Check sheet for the modelled part. Datum: model origin and axes. Units: mm. A direction names the side the tool comes from. Round coordinates to 2 decimals unless told otherwise and drop trailing zeros. Order: outer loops, then holes, each group sorted by start corner. A loop starts at its lowest first (then second) coordinate and runs counter-clockwise, first axis right, second up.
```python
from build123d import *

# Parameters (mm, degrees)
SKETCH1_W           = 26
SKETCH1_H           = 42
BOSS_EXTRUDE1_DEPTH = 16
SHELL1_T            = -2
SKETCH2_R           = 3.8
SKETCH2_R_2         = 1.8
BOSS_EXTRUDE2_DEPTH = 3
CUT_EXTRUDE2_START  = -2
SKETCH2_2_R         = 1.8
CUT_EXTRUDE2_DEPTH  = 2
SKETCH4_W           = 8
SKETCH4_H           = 10.725495138
CUT_EXTRUDE3_DEPTH  = 2
SKETCH5_W           = 6
SKETCH5_H           = 8.708980209
CUT_EXTRUDE4_DEPTH  = 2


with BuildPart() as part:
    # Sketch1 → Boss-Extrude1 (new body)
    with BuildSketch(Plane.XY):
        Rectangle(SKETCH1_W, SKETCH1_H)
    extrude(amount=BOSS_EXTRUDE1_DEPTH)

    # Shell1
    shell1_openings = [part.faces().sort_by_distance(p)[0] for p in [
        (0, 0, 16),
    ]]
    offset(amount=SHELL1_T, openings=shell1_openings, kind=Kind.INTERSECTION)

    # Sketch2 → Boss-Extrude2 (add)
    # profile 1 of 2: a face of its own
    with BuildSketch(Plane.XY.offset(2)):
        with Locations((-3.288169065, -4.006418736)):
            Circle(SKETCH2_R)
        with Locations((-3.288169065, -4.006418736)):
            Circle(SKETCH2_R_2, mode=Mode.SUBTRACT)
    # profile 2 of 2: a face of its own
    with BuildSketch(Plane.XY.offset(2)):
        with Locations((6.486240627, 13.735356113)):
            Circle(SKETCH2_R)
        with Locations((6.486240627, 13.735356113)):
            Circle(SKETCH2_R_2, mode=Mode.SUBTRACT)
    extrude(amount=BOSS_EXTRUDE2_DEPTH)

    # Sketch2<2> → Cut-Extrude2 (cut)
    with BuildSketch(Plane.XY.offset(2).offset(CUT_EXTRUDE2_START)):
        with Locations((6.486240627, 13.735356113)):
            Circle(SKETCH2_2_R)
        with Locations((-3.288169065, -4.006418736)):
            Circle(SKETCH2_2_R)
    extrude(amount=CUT_EXTRUDE2_DEPTH, mode=Mode.SUBTRACT)

    # Sketch4 → Cut-Extrude3 (cut)
    with BuildSketch(Plane.ZY.offset(13)):
        with Locations((10.6, 13.616095809)):
            Rectangle(SKETCH4_W, SKETCH4_H)
    extrude(amount=-CUT_EXTRUDE3_DEPTH, mode=Mode.SUBTRACT)

    # Sketch5 → Cut-Extrude4 (cut)
    with BuildSketch(Plane(origin=(13, 0, 0), x_dir=(0, 0, -1), z_dir=(1, 0, 0))):
        with Locations((-9.6, -14.594189668)):
            Rectangle(SKETCH5_W, SKETCH5_H)
    extrude(amount=-CUT_EXTRUDE4_DEPTH, mode=Mode.SUBTRACT)


solid = part.part
```
Item 1: Sectioned sample at D-D (y = 2). Record the cut outline in (x, z), and give its area (3 significant figures).
Answer:
outline: (-13, 0) - (13, 0) - (13, 16) - (11, 16) - (11, 2) - (-11, 2) - (-11, 16) - (-13, 16) - close
area: 108 mm2
Item 2: Sectioned sample at C-C (x = 5.5). Record the cut outline in (y, z), and give its area (3 significant figures).
Answer:
outline: (-21, 0) - (12.23, 0) - (12.23, 5) - (10.07, 5) - (10.07, 2) - (-19, 2) - (-19, 16) - (-21, 16) - close; (15.24, 0) - (21, 0) - (21, 16) - (19, 16) - (19, 2) - (17.41, 2) - (17.41, 5) - (15.24, 5) - close
area: 147 mm2
Item 3: Scan lines: line 1 along X through (y, z) = (-2, 7); line 2 along Y through (x, z) = (7.5, 7.25); line 3 along Y through (x, z) = (-11.75, 13.75). Record each from-to range of solid material in increasing order.
Answer:
line 1: x = -13 to -11, 11 to 13
line 2: y = -21 to -19, 19 to 21
line 3: y = -21 to 8.25, 18.98 to 21
Item 4: Access from +Z, -Z, +X, -X, +Y, -Y to the whole of each face (thin tool, end or side, straight path). Record for faces 1 (the flat face through (12, -18.949, 10)), 2 (the flat face through (0, 0, 2)), 3 (the flat face through (-12, 18.979, 11)), 4 (the flat face through (-13, -5, 8)).
Answer:
face 1: +X
face 2: +Z
face 3: -X
face 4: +Z, -Z, -X, +Y, -Y
Item 5: Release check for a two-part mould opening along X. For faces 5 (the cylindrical face through (-7.084, -3.839, 3.479)), 6 (the flat face through (13, 0, 8)), 7 (the flat face through (12, -10.24, 10)) record: released by +X, released by -X, zero draft, split by the parting line, or undercut.
Answer:
face 5: undercut
face 6: released by +X
face 7: zero draft
Item 6: Sectioned sample at A-A (y = -18). Record the cut outline in (x, z), and give its area (3 significant figures).
Answer:
outline: (-13, 0) - (13, 0) - (13, 6.6) - (11, 6.6) - (11, 2) - (-11, 2) - (-11, 16) - (-13, 16) - close; (11, 12.6) - (13, 12.6) - (13, 16) - (11, 16) - close
area: 96.0 mm2
Item 7: Go/stop test with flat-tipped pins: P1, Ø5, axis at x = -7.5, y = 14, coming from the +Z side; P2, Ø4.5, axis at x = -3.29, y = -4.01, coming from the +Z side. Record where each tip stops, or that it passes through.
Answer:
P1: stops at z = 2
P2: stops at z = 5
